The model under review builds one solid part; all positions refer to its coordinate system, in mm. A direction names the side the tool comes from. Give positions to 0.01 mm unless a question says otherwise; leave off trailing zeros. Loops run counter-clockwise (first coordinate to the right, second up) from the corner with the lowest first, then second, coordinate; pieces in that order, holes last. Notation, with made-up numbers: M 46.25,88 L 99.25,88 A22 cw 99.25,113 Z; hole C 12.25,-13 d4. An arc over 180 degrees is marked long. Return JSON: item names as keys, results as strings. Group by question number.
```python
from build123d import *

# Parameters (mm, degrees)
SKETCH_2_W          = 180
SKETCH_2_H          = 140
EXTRUDE_1_DEPTH     = 5
EXTRUDE_1_2_DEPTH   = 115
EXTRUDE_2_DEPTH     = 2
CUT_EXTRUDE_1_DEPTH = 140.5
SKETCH_6_R          = 6.5
CUT_EXTRUDE_2_DEPTH = 6
FILLET_1_R          = 10
CUT_EXTRUDE_3_REACH = 98.5


with BuildPart() as part:
    # Эскиз2 → Extrude 1 (new body)
    with BuildSketch(Plane(origin=(0, 0, 0), x_dir=(1, 0, 0), z_dir=(0, 1, 0))):
        Rectangle(SKETCH_2_W, SKETCH_2_H)
    extrude(amount=EXTRUDE_1_DEPTH)

    # Эскиз3 → Extrude 1 2 (add)
    with BuildSketch(Plane(origin=(0, 5, 0), x_dir=(1, 0, 0), z_dir=(0, 1, 0))):
        with BuildLine():
            Line((-45.5, -22.5), (-45.5, 21.5))
            ThreePointArc((-45.5, 21.5), (-45.207106781, 22.207106781), (-44.5, 22.5))
            Line((-44.5, 22.5), (44.5, 22.5))
            ThreePointArc((44.5, 22.5), (45.207106781, 22.207106781), (45.5, 21.5))
            Line((45.5, 21.5), (45.5, -22.5))
            Line((45.5, -22.5), (49.5, -22.5))
            Line((49.5, -22.5), (49.5, 21.5))
            ThreePointArc((49.5, 21.5), (48.035533906, 25.035533906), (44.5, 26.5))
            Line((44.5, 26.5), (-44.5, 26.5))
            ThreePointArc((-44.5, 26.5), (-48.035533906, 25.035533906), (-49.5, 21.5))
            Line((-49.5, 21.5), (-49.5, -22.5))
            Line((-49.5, -22.5), (-45.5, -22.5))
        make_face()
    extrude(amount=EXTRUDE_1_2_DEPTH)

    # Эскиз4 → Бобышка-Вытянуть2 (add, symmetric)
    with BuildSketch(Plane(origin=(0, 0, 0), x_dir=(0, 0, -1), z_dir=(1, 0, 0))):
        Polygon((26.5, 71.683956091), (65, 5), (26.5, 5), align=None)
    extrude(amount=EXTRUDE_2_DEPTH, both=True)

    # Эскиз5 → Вырез-Вытянуть1 (cut, through all)
    with BuildSketch(Plane(origin=(49.5, 0, 0), x_dir=(0, 0, -1), z_dir=(1, 0, 0))):
        with BuildLine():
            Line((5, 108), (5, 96))
            ThreePointArc((5, 96), (0, 91), (-5, 96))
            Line((-5, 96), (-5, 108))
            ThreePointArc((-5, 108), (0, 113), (5, 108))
        make_face()
        with BuildLine():
            Line((5, 29), (5, 17))
            ThreePointArc((5, 17), (0, 12), (-5, 17))
            Line((-5, 17), (-5, 29))
            ThreePointArc((-5, 29), (0, 34), (5, 29))
        make_face()
    extrude(amount=-CUT_EXTRUDE_1_DEPTH, mode=Mode.SUBTRACT)

    # Эскиз6 → Вырез-Вытянуть2 (cut, through all)
    with BuildSketch(Plane(origin=(0, 5, 0), x_dir=(1, 0, 0), z_dir=(0, 1, 0))):
        with Locations(Location((-75, 55, 0), (0, 0, 270))):  # turned: the seam where the file's is
            Circle(SKETCH_6_R)
        with Locations(Location((-75, -55, 0), (0, 0, 270))):  # turned: the seam where the file's is
            Circle(SKETCH_6_R)
        with Locations(Location((75, 55, 0), (0, 0, 270))):  # turned: the seam where the file's is
            Circle(SKETCH_6_R)
        with Locations(Location((75, -55, 0), (0, 0, 270))):  # turned: the seam where the file's is
            Circle(SKETCH_6_R)
    extrude(amount=-CUT_EXTRUDE_2_DEPTH, mode=Mode.SUBTRACT)

    # Скругление1
    fillet_1_edges = [part.edges().sort_by_distance(p)[0] for p in [
        (90, 2.5, 70),
        (-90, 2.5, 70),
        (-90, 2.5, -70),
        (90, 2.5, -70),
    ]]
    fillet(fillet_1_edges, radius=FILLET_1_R)

    # Эскиз8 → Вырез-Вытянуть3 (cut, up to next)
    with BuildSketch(Plane(origin=(0, 0, -26.5), x_dir=(-1, 0, 0), z_dir=(0, 0, -1)), mode=Mode.PRIVATE) as cut_extrude_3_sk1:
        with BuildLine():
            Line((-17.5, 108), (-17.5, 96))
            ThreePointArc((-17.5, 96), (-22.5, 91), (-27.5, 96))
            Line((-27.5, 96), (-27.5, 108))
            ThreePointArc((-27.5, 108), (-22.5, 113), (-17.5, 108))
        make_face()
    cut_extrude_3_tool1 = extrude(cut_extrude_3_sk1.sketch, amount=-CUT_EXTRUDE_3_REACH, mode=Mode.PRIVATE) & part.part
    add(cut_extrude_3_tool1.solids().sort_by_distance((22.5, 102, -26.5))[0], mode=Mode.SUBTRACT)
    # Эскиз8 → Вырез-Вытянуть3 (cut, up to next)
    with BuildSketch(Plane(origin=(0, 0, -26.5), x_dir=(-1, 0, 0), z_dir=(0, 0, -1)), mode=Mode.PRIVATE) as cut_extrude_3_sk2:
        with BuildLine():
            Line((-17.5, 29), (-17.5, 17))
            ThreePointArc((-17.5, 17), (-22.5, 12), (-27.5, 17))
            Line((-27.5, 17), (-27.5, 29))
            ThreePointArc((-27.5, 29), (-22.5, 34), (-17.5, 29))
        make_face()
    cut_extrude_3_tool2 = extrude(cut_extrude_3_sk2.sketch, amount=-CUT_EXTRUDE_3_REACH, mode=Mode.PRIVATE) & part.part
    add(cut_extrude_3_tool2.solids().sort_by_distance((22.5, 23, -26.5))[0], mode=Mode.SUBTRACT)
    # Эскиз8 → Вырез-Вытянуть3 (cut, up to next)
    with BuildSketch(Plane(origin=(0, 0, -26.5), x_dir=(-1, 0, 0), z_dir=(0, 0, -1)), mode=Mode.PRIVATE) as cut_extrude_3_sk3:
        with BuildLine():
            Line((17.5, 108), (17.5, 96))
            ThreePointArc((17.5, 96), (22.5, 91), (27.5, 96))
            Line((27.5, 96), (27.5, 108))
            ThreePointArc((27.5, 108), (22.5, 113), (17.5, 108))
        make_face()
    cut_extrude_3_tool3 = extrude(cut_extrude_3_sk3.sketch, amount=-CUT_EXTRUDE_3_REACH, mode=Mode.PRIVATE) & part.part
    add(cut_extrude_3_tool3.solids().sort_by_distance((-22.5, 102, -26.5))[0], mode=Mode.SUBTRACT)
    # Эскиз8 → Вырез-Вытянуть3 (cut, up to next)
    with BuildSketch(Plane(origin=(0, 0, -26.5), x_dir=(-1, 0, 0), z_dir=(0, 0, -1)), mode=Mode.PRIVATE) as cut_extrude_3_sk4:
        with BuildLine():
            Line((17.5, 29), (17.5, 17))
            ThreePointArc((17.5, 17), (22.5, 12), (27.5, 17))
            Line((27.5, 17), (27.5, 29))
            ThreePointArc((27.5, 29), (22.5, 34), (17.5, 29))
        make_face()
    cut_extrude_3_tool4 = extrude(cut_extrude_3_sk4.sketch, amount=-CUT_EXTRUDE_3_REACH, mode=Mode.PRIVATE) & part.part
    add(cut_extrude_3_tool4.solids().sort_by_distance((-22.5, 23, -26.5))[0], mode=Mode.SUBTRACT)


solid = part.part
```
(1) Add section A-A (z = 55). Write out the cut boundary in (x, y), and give its area (3 significant figures).
(2) For faces 1 (the flat face through (-45.5, 62, 1)), 2 (the cylindrical face through (-80.767, 2.535, 57.999)), 3 (the cylindrical face through (-47, 91, 0)), 4 (the flat face through (2, 24, -37)), 5 (the flat face through (17.5, 102, -25)), list the 3-axis set-ups (+Z, -Z, +X, -X, +Y, -Y) from which the entire face can be reached by the end or side of a thin tool; tool diameter is ignored.
(3) Add section C-C (x = 10.5). Write out the cut boundary in (y, z), and give its area (3 significant figures).
(4) For pin 1 (2 mm diameter, centred on x = -39, z = -35.5, fed in from +Y); pin 2 (1.2 mm diameter, centred on y = 23, z = -25, fed in from -X); pin 3 (1.2 mm diameter, centred on x = -47.5, y = 105, fed in from +Z), all flat-tipped, find the tip position at first contact; note any pin that passes through.
(5) Mouldability with a two-part tool opening along Z and no side actions: class faces 6 (the flat face through (-47, 102, 5)), 7 (the flat face through (-1, 2, 70)), 8 (the cylindrical face through (22.4, 91, -24.5)) as released by +Z, released by -Z, zero draft, split by the parting line, or undercut.
(6) Add section D-D (z = -45). Write out the cut boundary in (x, y).
(7) For probe 1 along X at (y, z) = (2.1, 55); probe 2 along X at (y, z) = (67.5, 6.5); probe 3 along Y at (x, z) = (4, 45), list the stretches that pass through material, from the lowest coordinate up.
(8) Add section B-B (y = 87). Write out the cut boundary in (x, z), and give its area (3 significant figures).
Verdict:
{
 "1": {"outline": "M -90,0 L -81.5,0 L -81.5,5 L -90,5 Z; M -68.5,0 L 68.5,0 L 68.5,5 L -68.5,5 Z; M 81.5,0 L 90,0 L 90,5 L 81.5,5 Z", "area": "770 mm²"},
 "2": {"face 1": "+Z, +Y", "face 2": "+Y, -Y", "face 3": "+X, -X", "face 4": "-Z, +X, +Y", "face 5": "+Z, -Z"},
 "3": {"outline": "M 0,-70 L 5,-70 L 5,-26.5 L 120,-26.5 L 120,-22.5 L 5,-22.5 L 5,70 L 0,70 Z", "area": "1,160 mm²"},
 "4": {"pin 1": "stops at y = 5", "pin 2": "stops at x = -48.57", "pin 3": "stops at z = 22.5"},
 "5": {"face 6": "undercut", "face 7": "released by +Z", "face 8": "zero draft"},
 "6": {"outline": "M -90,0 L 90,0 L 90,5 L 2,5 L 2,39.64 L -2,39.64 L -2,5 L -90,5 Z"},
 "7": {"probe 1": "x = -90 to -81.5, -68.5 to 68.5, 81.5 to 90", "probe 2": "x = -49.5 to -45.5, 45.5 to 49.5", "probe 3": "y = 0 to 5"},
 "8": {"outline": "M -49.5,-21.5 A5 ccw -44.5,-26.5 L 44.5,-26.5 A5 ccw 49.5,-21.5 L 49.5,22.5 L 45.5,22.5 L 45.5,-21.5 A1 cw 44.5,-22.5 L -44.5,-22.5 A1 cw -45.5,-21.5 L -45.5,22.5 L -49.5,22.5 Z", "area": "746 mm²"}
}
